from build123d import *

# Parameters (mm, degrees)
F0_R     = 1.75
F1_DEPTH = 4


with BuildPart() as f1:
    # F0 (on Top) → F1 (new body)
    with BuildSketch(Plane.XY):
        Polygon((23.22716, 3.353091), (3.22716, 3.353091), (3.22716, -14.646909), (10.551348, -14.646909), (16.259164, -8.379568), (23.22716, -8.379568), align=None)
        with Locations((7.22716, -10.646909)):
            Circle(F0_R, mode=Mode.SUBTRACT)
        with Locations((10.72716, -0.646909)):
            Circle(F0_R, mode=Mode.SUBTRACT)
        Polygon((43.22716, 3.353091), (23.22716, 3.353091), (23.22716, -8.379568), (30.195156, -8.379568), (35.902971, -14.646909), (43.22716, -14.646909), align=None)
        with Locations((39.22716, -10.646909)):
            Circle(F0_R, mode=Mode.SUBTRACT)
        with Locations((35.72716, -0.646909)):
            Circle(F0_R, mode=Mode.SUBTRACT)
    extrude(amount=F1_DEPTH)


solid = f1.part
The listing builds one solid part. Answer for the finished solid, in the listing's coordinates (mm). A direction names the side the tool comes from. Round coordinates to 2 decimals unless told otherwise and drop trailing zeros. Write each loop counter-clockwise with the first axis right and the second up, starting at its lowest first coordinate (ties: lowest second). Pieces come first, ordered by that corner, then holes. Notation, with made-up numbers: M 89.5,22.25 L 124.5,22.25 A13 ccw 124.5,27.25 Z; hole C 49,5.5 d10. An arc over 180 degrees is marked long. Write each question's results on one line, items separated by ' | '. Start each with the question number.
Item 1: Given pin 1 Ø8 at (x, y) = (38, -10.5) entering from -Z; pin 2 Ø3 at (x, y) = (16, -11) entering from -Z; pin 3 Ø2 at (x, z) = (20.5, 3) entering from -Y, each flat-ended and moving along its own axis, determine where each tip first touches the part or whether it passes through.
Item 2: Find section A-A on x = 11. Write down the section's boundary in (y, z), and give its area (3 significant figures).
Item 3: Find section D-D on y = -10. Write down the section's boundary in (x, z), and give its area (3 significant figures).
Item 4: Find section C-C on z = 0.8. Write down the section's boundary in (x, y), and give its area (3 significant figures).
Item 5: Straight lines are drawn through the part: probe 1 along X at (y, z) = (-0.75, 0.6); probe 2 along X at (y, z) = (-1.25, 1); probe 3 along Y at (x, z) = (18.5, 0.7). For each, find the intervals that lie inside material, in ascending order.
Item 6: Find section B-B on y = -13.25. Write down the section's boundary in (x, z), and give its area (3 significant figures).
Item 7: Which of the six approach directions +Z, -Z, +X, -X, +Y, -Y give full straight-line access (tool end or side, diameter ignored) to faces 5 (the cylindrical face through (7, -8.91, 1.97)), 6 (the flat face through (23, -8.38, 2))?
Item 8: The mould has two halves that part along Y. Classify faces 1 (the cylindrical face through (40.896, -10.121, 1.972)), 2 (the cylindrical face through (12.396, -0.121, 1.972)), 3 (the flat face through (7, -14.647, 2)), 4 (the flat face through (24, 3.353, 2)): +Y half, -Y half, draft (parallel to the pull), parting line (faces both ways), or undercut.
Answer block:
1) pin 1: stops at z = 0 | pin 2: passes through | pin 3: stops at y = -8.38
2) outline: M -14.15,0 L -2.38,0 L -2.38,4 L -14.15,4 Z; M 1.08,0 L 3.35,0 L 3.35,4 L 1.08,4 Z | area: 56.2 mm²
3) outline: M 3.23,0 L 5.6,0 L 5.6,4 L 3.23,4 Z; M 8.85,0 L 14.78,0 L 14.78,4 L 8.85,4 Z; M 31.67,0 L 37.6,0 L 37.6,4 L 31.67,4 Z; M 40.85,0 L 43.23,0 L 43.23,4 L 40.85,4 Z | area: 66.4 mm²
4) outline: M 3.23,-14.65 L 10.55,-14.65 L 16.26,-8.38 L 30.2,-8.38 L 35.9,-14.65 L 43.23,-14.65 L 43.23,3.35 L 3.23,3.35 Z; hole C 7.23,-10.65 d3.5; hole C 10.73,-0.65 d3.5; hole C 35.73,-0.65 d3.5; hole C 39.23,-10.65 d3.5 | area: 558 mm²
5) probe 1: x = 3.23 to 8.98, 12.47 to 33.98, 37.47 to 43.23 | probe 2: x = 3.23 to 9.08, 12.37 to 34.08, 37.37 to 43.23 | probe 3: y = -8.38 to 3.35
6) outline: M 3.23,0 L 11.82,0 L 11.82,4 L 3.23,4 Z; M 34.63,0 L 43.23,0 L 43.23,4 L 34.63,4 Z | area: 68.8 mm²
7) face 5: +Z, -Z | face 6: +Z, -Z, -Y
8) face 1: undercut | face 2: undercut | face 3: -Y half | face 4: +Y half
